Input: dimensioned drawing with shaded views. Units: mm. Origin: part minimum x, y, z. Round coordinates to 2 decimals unless told otherwise and drop trailing zeros. Loops run counter-clockwise (first coordinate to the right, second up) from the corner with the lowest first, then second, coordinate; pieces in that order, holes last. Notation, with made-up numbers: (19.5, 15) - (73.5, 15) arc R16 cw to (73.5, 36) - close; hole circle Ø2 at (71, -33.75). An arc over 180 degrees is marked (long way). Use CSV: the item, a comma, the result in double quotes. Start each with the question number.
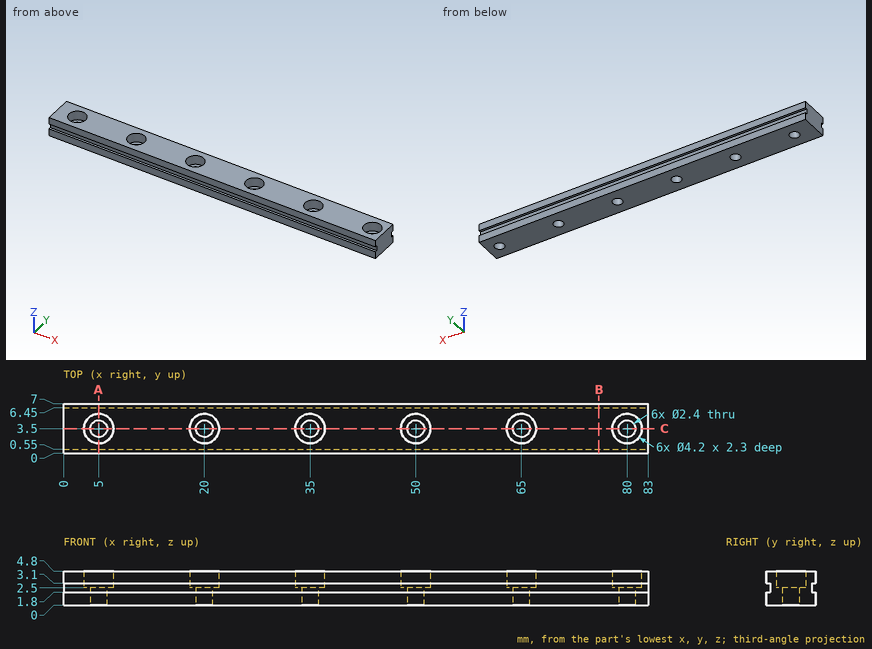
1. Section query C-C on y = 3.5. Give the number of separate pieces and of enclosed holes in the cut face, and give its area (3 significant figures).
2. Contact query for flat-ended pins moving along their axis: P1, Ø1.4, axis at x = 80, y = 3.5, coming from the -Z side; P2, Ø4, axis at x = 35, y = 3.5, coming from the +Z side; P3, Ø0.6, axis at x = 40.5, z = 2.5, coming from the +Y side; P4, Ø0.6, axis at x = 61.5, z = 2.5, coming from the -Y side. Output: stop coordinate, or through.
3. Section query B-B on x = 76. Return the cut outline in (y, z).
4. Line query: line 1 along Y through (x, z) = (20, 1.05); line 2 along Z through (x, y) = (72, 6.5); line 3 along Y through (x, z) = (35, 3.85). Output: solid intervals per line, ascending.
5. Section query A-A on x = 5. Return the cut outline in (y, z).
Values:
1,separate pieces,"7"
1,enclosed holes,"0"
1,area,"304 mm^2"
2,P1,"passes through"
2,P2,"stops at z = 2.5"
2,P3,"stops at y = 6.45"
2,P4,"stops at y = 0.55"
3,outline,"(0, 0) - (7, 0) - (7, 1.8) - (6.45, 1.8) - (6.45, 3.1) - (7, 3.1) - (7, 4.8) - (0, 4.8) - (0, 3.1) - (0.55, 3.1) - (0.55, 1.8) - (0, 1.8) - close"
4,line 1,"y = 0 to 2.3, 4.7 to 7"
4,line 2,"z = 0 to 1.8, 3.1 to 4.8"
4,line 3,"y = 0 to 1.4, 5.6 to 7"
5,outline,"(0, 0) - (2.3, 0) - (2.3, 2.5) - (1.4, 2.5) - (1.4, 4.8) - (0, 4.8) - (0, 3.1) - (0.55, 3.1) - (0.55, 1.8) - (0, 1.8) - close; (4.7, 0) - (7, 0) - (7, 1.8) - (6.45, 1.8) - (6.45, 3.1) - (7, 3.1) - (7, 4.8) - (5.6, 4.8) - (5.6, 2.5) - (4.7, 2.5) - close"
